Read the model definition and answer for the solid it produces. Units are mm, in the model's axes. A direction names the side the tool comes from. Coordinates: 2 decimals unless noted, no trailing zeros. Loops run counter-clockwise (first coordinate to the right, second up) from the corner with the lowest first, then second, coordinate; pieces in that order, holes last.
Q1. Which of the six approach directions +Z, -Z, +X, -X, +Y, -Y give full straight-line access (tool end or side, diameter ignored) to faces 5 (the face through (0.711, 127.454, 32.017)), 6 (the face through (50.8, 51, 1)), 7 (the face through (41.275, 60, 0))?
Q2. Section A-A (x = -30.5) is taken. Give the vertices of the cut face in (y, z) (3 decimals).
Q3. Section D-D (y = 117.5) is taken. Give the vertices of the cut face in (x, z) (3 decimals), then the cut area to 3 significant figures.
Q4. Section C-C (z = 6) is taken. Give the vertices of the cut face in (x, y) (3 decimals), then the cut area to 3 significant figures.
Q5. Section B-B (y = 64) is taken. Give the vertices of the cut face in (x, z) (3 decimals), then the cut area to 3 significant figures.
Q6. Straight lines are drawn through the part: line 1 (X direction, y = 40, z = -7) (3 decimals); line 2 (Z direction, x = -26.5, y = 21) (3 decimals); line 3 (Y direction, x = -22.5, z = -33). For each, find the intervals that lie inside material, in ascending order.
Q7. The mould has two halves that part along X. Classify faces 1 (the face through (40.32, 61.14, 27.67)), 2 (the face through (0.711, 126.92, -31.483)), 3 (the face through (-40.32, 61.14, -27.67)), 4 (the face through (-50.8, 51, -1)): pulls with the +X half, pulls with the -X half, needs draft (parallel to the pull), parting line crosses it, or undercut.
from build123d import *

# Parameters (mm, degrees)
BOSS_EXTRUDE1_DEPTH = 508
CUT_EXTRUDE7_REACH  = 521.459


with BuildPart() as part:
    # Sketch1 → Boss-Extrude1 (new body)
    with BuildSketch(Plane(origin=(0, 0, 0), x_dir=(1, 0, 0), z_dir=(0, 1, 0))):
        Polygon((-52.613166046, -38.1), (52.613166046, -38.1), (50.8, -38.1), (50.8, -0.977324315), (50.8, 0.977324315), (50.8, 38.1), (39.913166046, 38.1), (-39.913166046, 38.1), (-50.8, 38.1), (-50.8, -24.422675685), (-50.8, 24.422675685), (-50.8, -38.1), align=None)
        with BuildLine():
            Line((-38.1, -28.575), (38.1, -28.575))
            ThreePointArc((38.1, -28.575), (40.34506403, -27.64506403), (41.275, -25.4))
            Line((41.275, -25.4), (41.275, 25.4))
            ThreePointArc((41.275, 25.4), (40.34506403, 27.64506403), (38.1, 28.575))
            Line((38.1, 28.575), (-38.1, 28.575))
            ThreePointArc((-38.1, 28.575), (-40.34506403, 27.64506403), (-41.275, 25.4))
            Line((-41.275, 25.4), (-41.275, -25.4))
            ThreePointArc((-41.275, -25.4), (-40.34506403, -27.64506403), (-38.1, -28.575))
        make_face(mode=Mode.SUBTRACT)
    extrude(amount=BOSS_EXTRUDE1_DEPTH)

    # Cut-Extrude7: up to this face of the body (flat: up to its plane)
    cut_extrude7_end = Plane(part.part.faces().sort_by_distance((-50.8, 254, 0))[0])
    # Sketch8 → Cut-Extrude7 (cut, up to the picked face)
    with BuildSketch(Plane(origin=(50.8, 0, 0), x_dir=(0, 0, -1), z_dir=(1, 0, 0)), mode=Mode.PRIVATE) as cut_extrude7_sk1:
        Polygon((-38.1, 133.5369186), (0, 95.4369186), (38.1, 133.5369186), (38.1, 508), (-38.1, 508), align=None)
    cut_extrude7_tool1 = split(extrude(cut_extrude7_sk1.sketch, amount=-CUT_EXTRUDE7_REACH, mode=Mode.PRIVATE), bisect_by=cut_extrude7_end, keep=Keep.BOTH, mode=Mode.PRIVATE)
    add(cut_extrude7_tool1.solids().sort_by(Axis((50.8, 311.089757, 0), (-1, 0, 0)))[0], mode=Mode.SUBTRACT)


solid = part.part
Numbers:
1. face 5: +X, -X, +Y
1. face 6: +Z, -Z, +X, +Y, -Y
1. face 7: +Y, -Y
2. outline: (0, -38.1) - (133.537, -38.1) - (124.012, -28.575) - (0, -28.575) - close; (0, 28.575) - (124.012, 28.575) - (133.537, 38.1) - (0, 38.1) - close
3. outline: (-50.8, -38.1) - (50.8, -38.1) - (50.8, -22.063) - (41.275, -22.063) - (41.275, -25.4) arc R3.175 cw to (38.1, -28.575) - (-38.1, -28.575) arc R3.175 cw to (-41.275, -25.4) - (-41.275, -22.063) - (-50.8, -22.063) - close; (-50.8, 22.063) - (-41.275, 22.063) - (-41.275, 25.4) arc R3.175 cw to (-38.1, 28.575) - (38.1, 28.575) arc R3.175 cw to (41.275, 25.4) - (41.275, 22.063) - (50.8, 22.063) - (50.8, 38.1) - (-50.8, 38.1) - close
3. area: 2,190 mm2
4. outline: (-50.8, 0) - (-41.275, 0) - (-41.275, 101.437) - (-50.8, 101.437) - close; (41.275, 0) - (50.8, 0) - (50.8, 101.437) - (41.275, 101.437) - close
4. area: 1,930 mm2
5. outline: (-50.8, -38.1) - (50.8, -38.1) - (50.8, 38.1) - (-50.8, 38.1) - close; hole (-41.275, -25.4) arc R3.175 ccw to (-38.1, -28.575) - (38.1, -28.575) arc R3.175 ccw to (41.275, -25.4) - (41.275, 25.4) arc R3.175 ccw to (38.1, 28.575) - (-38.1, 28.575) arc R3.175 ccw to (-41.275, 25.4) - close
5. area: 3,030 mm2
6. line 1: x = -50.8 to -41.275, 41.275 to 50.8
6. line 2: z = -38.1 to -28.575, 28.575 to 38.1
6. line 3: y = 0 to 128.44
7. face 1: undercut
7. face 2: needs draft
7. face 3: undercut
7. face 4: pulls with the -X half
